For this review, take the finished solid that the model builds, in its own axes (mm). Face numbers are marked on the shaded views. Give positions to 0.01 mm unless a question says otherwise; leave off trailing zeros. Answer as CSV lines item,"result". Start each with the question number.
1. Mouldability with a two-part tool opening along X and no side actions: class the marked faces 1 and 2 as pulls with the +X half, pulls with the -X half, needs draft (parallel to the pull), parting line crosses it, or undercut.
2. Clearance check with flat-ended pins moving along their axes: P1, Ø3, axis at y = -26.99, z = -46.74, coming from the +X side; P2, Ø2, axis at x = -43, z = 5, coming from the +Y side; P3, Ø5.5, axis at y = -53.975, z = 0, coming from the +X side; P4, Ø3, axis at y = 37, z = -1.5, coming from the +X side. State where each tip first meets the part, or that it passes through.
3. For line 1 along Y through (x, z) = (0.35, 0); line 2 along X through (y, z) = (-33, 46); line 3 along Y through (x, z) = (-9, -8), list the stretches that pass through material, from the lowest coordinate up.
Autodesk Inventor part; units mm, degrees
ref_plane "YZ Plane" through (0, 0, 0) normal (1, 0, 0) x (0, 1, 0)
ref_plane "XZ Plane" through (0, 0, 0) normal (0, 1, 0) x (-1, 0, 0)
ref_plane "XY Plane" through (0, 0, 0) normal (0, 0, 1) x (1, 0, 0)
sketch "Sketch1" plane through (0, 0, 0) normal (0, 1, 0) x (-1, 0, 0)
  arc A0 (50.8, 0) -> (1.2863, 50.7837) centre (0, 0) ccw
  line L0 (1.2863, 50.7837) -> (1.2863, 57.15)
  line L1 (-1.2537, 57.15) -> (-1.2537, 48.2437)
  arc A1 (48.26, 0) -> (-1.2537, 48.2437) centre (0, 0) ccw
  line L2 (1.2863, 57.15) -> (-1.2537, 57.15)
  line L3 (50.8, 0) -> (48.2557, 0)
  dimension "d0" = 50.8
  dimension "d5" = 2.54
  dimension "d19" = 57.15
revolve "Revolution1" add sketch "Sketch1" angle 360 about axis through (-50.8, 0, 0) along (1, 0, 0)
sketch "Sketch2" plane through (-1.2863, 0, 0) normal (-1, 0, 0) x (0, 0, 1)
  circle A0 centre (0, 53.975) radius 1.7526
  circle A1 centre (0, 0) radius 50.7837
  circle A2 centre (-46.7437, 26.9875) radius 1.7526
  circle A3 centre (-46.7437, -26.9875) radius 1.7526
  circle A4 centre (0, -53.975) radius 1.7526
  circle A5 centre (46.7437, -26.9875) radius 1.7526
  circle A6 centre (46.7437, 26.9875) radius 1.7526
  dimension "d10" = 3.5052
  dimension "d12" = 53.975
  dimension "d15" = 360
extrude "Extrusion1" cut sketch "Sketch2" against normal blind 254 contours A0 | A2 | A3 | A4 | A5 | A6
properties part number "ROV Dome 4''"
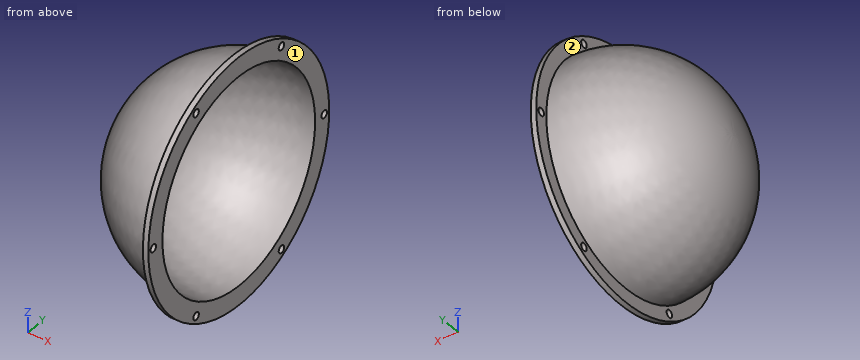
Result set:
1,face 1,"pulls with the +X half"
1,face 2,"pulls with the -X half"
2,P1,"through"
2,P2,"y = 28.15"
2,P3,"x = 1.25"
2,P4,"x = -29.06"
3,line 1,"-57.15 to -55.73, -52.22 to -48.26, 48.26 to 52.22, 55.73 to 57.15"
3,line 2,"-1.29 to 1.25"
3,line 3,"-49.35 to -46.73, 46.73 to 49.35"
